CAD build for the part. Positions are in the model's coordinates, mm. A direction names the side the tool comes from. Round coordinates to 2 decimals unless told otherwise and drop trailing zeros. Loops run counter-clockwise (first coordinate to the right, second up) from the corner with the lowest first, then second, coordinate; pieces in that order, holes last.
Autodesk Inventor part; units mm, degrees
ref_plane "YZ Plane" through (0, 0, 0) normal (1, 0, 0) x (0, 1, 0)
ref_plane "XZ Plane" through (0, 0, 0) normal (0, 1, 0) x (-1, 0, 0)
ref_plane "XY Plane" through (0, 0, 0) normal (0, 0, 1) x (1, 0, 0)
sketch "Sketch1" plane through (0, 0, 0) normal (0, 1, 0) x (-1, 0, 0)
  line L0 (-22.01, 11.46) -> (22.01, 11.46)
  line L1 (22.01, 11.46) -> (22.01, -11.46)
  line L2 (22.01, -11.46) -> (-22.01, -11.46)
  line L3 (-22.01, -11.46) -> (-22.01, 11.46)
  line L4 (-22.01, 11.46) -> (22.01, -11.46) construction
  line L5 (22.01, 11.46) -> (-22.01, -11.46) construction
  line L6 (20.1, -9.1) -> (-20.1, -9.1) construction
  line L7 (-20.1, -9.1) -> (-20.1, 9.1) construction
  line L8 (-20.1, 9.1) -> (20.1, 9.1) construction
  line L9 (20.1, 9.1) -> (20.1, -9.1) construction
  line L10 (20.1, -9.1) -> (-20.1, 9.1) construction
  line L11 (-20.1, -9.1) -> (20.1, 9.1) construction
  circle A0 centre (11.35, 0) radius 5.08
  point P0 (0, 0)
  point P1 (22.01, 0)
  dimension "d0" = 18.2
  dimension "d1" = 40.2
  dimension "d2" = 44.02
  dimension "d3" = 22.92
  dimension "d4" = 33.36
  dimension "d5" = 10.16
extrude "Extrusion1" add sketch "Sketch1" along normal mid plane 27 contours L0 L1 L2 L3 | A0
hole "Hole1" at (20.1, 0, -9.1) at (20.1, 0, 9.1) at (-20.1, 0, -9.1) at (-20.1, 0, 9.1) direction (0, 1, 0) diameter 2.5 end through all both
chamfer "Chamfer1" distance 0.5 angle 45 4 edges at (-22.01, 0, -11.46) (-22.01, 0, 11.46) (22.01, 0, -11.46) (22.01, 0, 11.46)
extrude "Extrusion2" add sketch "Sketch1" along normal mid plane 32.12 contours A0
properties part number "Servo_Block"
Item 1: Cut at B-B (y = -3.5). List the corners of the cut face in (x, z), plus the area to 3 significant figures.
Verdict:
outline: (-22.01, -10.96) - (-21.51, -11.46) - (21.51, -11.46) - (22.01, -10.96) - (22.01, 10.96) - (21.51, 11.46) - (-21.51, 11.46) - (-22.01, 10.96) - close; hole circle Ø2.5 at (-20.1, -9.1); hole circle Ø2.5 at (-20.1, 9.1); hole circle Ø2.5 at (20.1, -9.1); hole circle Ø2.5 at (20.1, 9.1)
area: 989 mm2
Item 2: Flat gauge pins, fed straight in: P1, Ø8, axis at x = 7, z = -4.5, coming from the +Y side; P2, Ø1.5, axis at x = -20.1, z = -9.1, coming from the +Y side; P3, Ø10, axis at x = -12.5, z = 5, coming from the -Y side; P4, Ø2, axis at x = -17, z = 3, coming from the -Y side. Where does each tip first touch, or does it go through?
Verdict:
P1: stops at y = 13.5
P2: passes through
P3: stops at y = -16.06
P4: stops at y = -13.5
Item 3: Cut at C-C (z = -9.1). List the corners of the cut face in (x, y).
Verdict:
outline: (-22.01, -13.5) - (-21.35, -13.5) - (-21.35, 13.5) - (-22.01, 13.5) - close; (-18.85, -13.5) - (18.85, -13.5) - (18.85, 13.5) - (-18.85, 13.5) - close; (21.35, -13.5) - (22.01, -13.5) - (22.01, 13.5) - (21.35, 13.5) - close
Item 4: Wall check: L1, parallel to Z at x = 20.1, y = 5.5; L2, parallel to X at y = -1, z = 9; L3, parallel to X at y = 3, z = -8.25. Give the ranges that are in metal, low to high.
Verdict:
L1: z = -11.46 to -10.35, -7.85 to 7.85, 10.35 to 11.46
L2: x = -22.01 to -21.35, -18.85 to 18.85, 21.35 to 22.01
L3: x = -22.01 to -21.02, -19.18 to 19.18, 21.02 to 22.01
Item 5: 3-axis set-ups, long thin cutter, end or side, ignore diameter. For faces 1 (the cylindrical face through (-16.195, -14.762, 1.526)), 2 (the flat face through (22.01, 0, 0)): which of +Z, -Z, +X, -X, +Y, -Y reach the whole face in a straight line?
Verdict:
face 1: -Y
face 2: +Z, -Z, +X, +Y, -Y
Item 6: Cut at D-D (x = -11.35). List the corners of the cut face in (y, z).
Verdict:
outline: (-16.06, -5.08) - (-13.5, -5.08) - (-13.5, -11.46) - (13.5, -11.46) - (13.5, -5.08) - (16.06, -5.08) - (16.06, 5.08) - (13.5, 5.08) - (13.5, 11.46) - (-13.5, 11.46) - (-13.5, 5.08) - (-16.06, 5.08) - close
Item 7: Cut at A-A (x = -20.1). List the corners of the cut face in (y, z), plus the area to 3 significant figures.
Verdict:
outline: (-13.5, -11.46) - (13.5, -11.46) - (13.5, -10.35) - (-13.5, -10.35) - close; (-13.5, -7.85) - (13.5, -7.85) - (13.5, 7.85) - (-13.5, 7.85) - close; (-13.5, 10.35) - (13.5, 10.35) - (13.5, 11.46) - (-13.5, 11.46) - close
area: 484 mm2
Item 8: Mould opens along Z. For faces 3 (the cylindrical face through (-21.154, 0.189, -9.772)), 4 (the flat face through (-22.01, 0, 0)), 5 (the cylindrical face through (-16.195, 14.762, -1.526)), 6 (the flat face through (0, 0, -11.46)) say: released by +Z, released by -Z, zero draft, split by the parting line, or undercut.
Verdict:
face 3: undercut
face 4: zero draft
face 5: split by the parting line
face 6: released by -Z
